The listing builds one solid part. Answer for the finished solid, in the listing's coordinates (mm). A direction names the side the tool comes from. Give positions to 0.01 mm unless a question says otherwise; leave off trailing zeros. Write each loop counter-clockwise with the first axis right and the second up, starting at its lowest first coordinate (ties: lowest second). Pieces come first, ordered by that corner, then holes.
```python
from build123d import *

# Parameters (mm, degrees)
SKETCH1_R           = 18.5
BOSS_EXTRUDE1_DEPTH = 25
SKETCH2_R           = 6
BOSS_EXTRUDE2_DEPTH = 6.8
SKETCH3_R           = 3
BOSS_EXTRUDE3_DEPTH = 20
SKETCH5_R           = 13.7
BOSS_EXTRUDE4_DEPTH = 25


with BuildPart() as part:
    # Sketch1 → Boss-Extrude1 (new body)
    with BuildSketch(Plane.XY):
        Circle(SKETCH1_R)
    extrude(amount=BOSS_EXTRUDE1_DEPTH)

    # Sketch2 → Boss-Extrude2 (add)
    with BuildSketch(Plane(origin=(0, 0, 0), x_dir=(-1, 0, 0), z_dir=(0, 0, -1))):
        Circle(SKETCH2_R)
    extrude(amount=BOSS_EXTRUDE2_DEPTH)

    # Sketch3 → Boss-Extrude3 (add)
    with BuildSketch(Plane(origin=(0, 0, -6.8), x_dir=(-1, 0, 0), z_dir=(0, 0, -1))):
        Circle(SKETCH3_R)
    extrude(amount=BOSS_EXTRUDE3_DEPTH)

    # Sketch5 → Boss-Extrude4 (add)
    with BuildSketch(Plane.XY.offset(25)):
        Circle(SKETCH5_R)
    extrude(amount=BOSS_EXTRUDE4_DEPTH)


solid = part.part
```
Item 1: A cutting plane is placed at A-A, the plane y = 0. Give the vertices of the cut face in (x, z), plus the area to 3 significant figures.
Conclusion:
outline: (-18.5, 0) - (-6, 0) - (-6, -6.8) - (-3, -6.8) - (-3, -26.8) - (3, -26.8) - (3, -6.8) - (6, -6.8) - (6, 0) - (18.5, 0) - (18.5, 25) - (13.7, 25) - (13.7, 50) - (-13.7, 50) - (-13.7, 25) - (-18.5, 25) - close
area: 1,810 mm2
Item 2: A cutting plane is placed at C-C, the plane z = -14.5. Give the vertices of the cut face in (x, y), plus the area to 3 significant figures.
Conclusion:
outline: circle Ø6 at (0, 0)
area: 28.3 mm2
Item 3: Consider probe 1 along Z at (x, y) = (-5, -8); probe 2 along Z at (x, y) = (15.5, -3); probe 3 along Y at (x, z) = (0, 6). Determine where each line is inside the solid, lowest interval first.
Conclusion:
probe 1: z = 0 to 50
probe 2: z = 0 to 25
probe 3: y = -18.5 to 18.5
Item 4: A cutting plane is placed at D-D, the plane x = -8. Give the vertices of the cut face in (y, z), plus the area to 3 significant figures.
Conclusion:
outline: (-16.68, 0) - (16.68, 0) - (16.68, 25) - (11.12, 25) - (11.12, 50) - (-11.12, 50) - (-11.12, 25) - (-16.68, 25) - close
area: 1,390 mm2
Item 5: Each of these flat-tipped pins is pushed along its axis until it touches: P1, Ø12, axis at y = 1.5, z = -17, coming from the +X side; P2, Ø1, axis at y = 2.5, z = 21, coming from the +X side; P3, Ø8, axis at y = -14.5, z = 21.5, coming from the -X side. Where does it stop, or does it pass through?
Conclusion:
P1: stops at x = 3
P2: stops at x = 18.39
P3: stops at x = -15.23
Item 6: Which of the six approach directions +Z, -Z, +X, -X, +Y, -Y give full straight-line access (tool end or side, diameter ignored) to faces 1 (the face through (3, 0, -17)), 2 (the face through (-10.097, 9.259, 37.325)), 3 (the face through (0, 0, -26.8))?
Conclusion:
face 1: -Z
face 2: +Z
face 3: -Z, +X, -X, +Y, -Y
